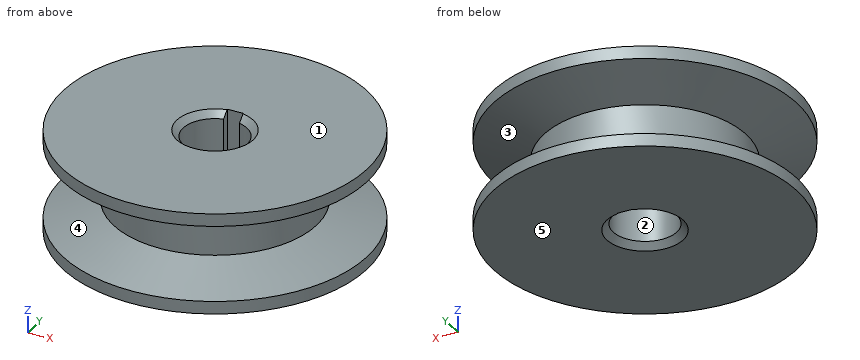
```python
from build123d import *

# Parameters (mm, degrees)
SKETCH1_R          = 19.05
SKETCH1_R_2        = 4
EXTRUDE1_DEPTH     = 6.35
CHAMFER1_SIZE      = 0.79375
SKETCH3_W          = 2
SKETCH3_H          = 2
CUT_EXTRUDE1_DEPTH = 30.784140075


with BuildPart() as part:
    # Sketch1 → Extrude1 (new, symmetric)
    with BuildSketch(Plane.XY):
        Circle(SKETCH1_R)
        Circle(SKETCH1_R_2, mode=Mode.SUBTRACT)
    extrude(amount=EXTRUDE1_DEPTH, both=True)

    # Chamfer1
    chamfer1_edges = [part.edges().sort_by_distance(p)[0] for p in [
        (-4, 0, -6.35),
        (-4, 0, 6.35),
    ]]
    chamfer(chamfer1_edges, length=CHAMFER1_SIZE)

    # Sketch2 → Cut-Revolve1 (revolve, cut)
    with BuildSketch(Plane(origin=(0, 0, 0), x_dir=(0, 0, -1), z_dir=(1, 0, 0)), mode=Mode.PRIVATE) as cut_revolve1_sk:
        Polygon((-4.7625, 19.05), (4.7625, 19.05), (2.451289012, 12.7), (-2.451289012, 12.7), align=None)
    revolve(cut_revolve1_sk.sketch.rotate(Axis((0, 0, 6.35), (0, 0, -1)), 180), axis=Axis((0, 0, 6.35), (0, 0, -1)), mode=Mode.SUBTRACT)

    # Sketch3 → Cut-Extrude1 (cut, through all)
    with BuildSketch(Plane.XY.offset(6.35)):
        with Locations((0, 3.8)):
            Rectangle(SKETCH3_W, SKETCH3_H)
    extrude(amount=-CUT_EXTRUDE1_DEPTH, mode=Mode.SUBTRACT)


solid = part.part
```
The model under review builds one solid part; all positions refer to its coordinate system, in mm. Face numbers are marked on the shaded views. A direction names the side the tool comes from. Give positions to 0.01 mm unless a question says otherwise; leave off trailing zeros. Write each loop counter-clockwise with the first axis right and the second up, starting at its lowest first coordinate (ties: lowest second). Pieces come first, ordered by that corner, then holes.
(1) Tool access review of the marked faces 4 and 5: name each direction out of +Z, -Z, +X, -X, +Y, -Y from which nothing blocks a thin tool from reaching the whole face with its end or side.
(2) For P1, Ø3, axis at y = -9.5, z = 0, coming from the -X side; P2, Ø2, axis at x = -0.5, z = 0.5, coming from the -Y side; P3, Ø5, axis at y = 4, z = 3.5, coming from the +X side; P4, Ø6.5, axis at x = 0, y = 0, coming from the -Z side, all flat-tipped, find the tip position at first contact; note any pin that passes through.
(3) To check wall thickness, follow L1, parallel to X at y = 0, z = 0.75; L2, parallel to Z at x = -3, y = 16.5; L3, parallel to Y at x = 2, z = -0.75. State the ranges of each line that lie inside material, in increasing order.
(4) Consider section C-C, the plane z = 0.75. Give the boundary of the cut face in (x, y).
(5) The part is to be moulded in two halves that separate along X. For the marked faces 1, 2 and 3, say which applies: released by +X, released by -X, zero draft, split by the parting line, or undercut.
(6) Consider section A-A, the plane y = 0. Give the boundary of the cut face in (x, z).
(7) Consider section B-B, the plane x = 0. Give the boundary of the cut face in (y, z), and give its area (3 significant figures).
Returned:
1. face 4: none
1. face 5: -Z, +X, -X, +Y, -Y
2. P1: stops at x = -9.86
2. P2: stops at y = -12.7
2. P3: stops at x = 18.96
2. P4: passes through
3. L1: x = -12.7 to -4, 4 to 12.7
3. L2: z = -6.35 to -3.93, 3.93 to 6.35
3. L3: y = -12.54 to -3.46, 3.46 to 12.54
4. outline: circle Ø25.4 at (0, 0); hole (-1, 3.87) arc R4 ccw (long way) to (1, 3.87) - (1, 4.8) - (-1, 4.8) - close
5. face 1: zero draft
5. face 2: undercut
5. face 3: split by the parting line
6. outline: (-19.05, -6.35) - (-4.79, -6.35) - (-4, -5.56) - (-4, 5.56) - (-4.79, 6.35) - (-19.05, 6.35) - (-19.05, 4.76) - (-12.7, 2.45) - (-12.7, -2.45) - (-19.05, -4.76) - close; (4, -5.56) - (4.79, -6.35) - (19.05, -6.35) - (19.05, -4.76) - (12.7, -2.45) - (12.7, 2.45) - (19.05, 4.76) - (19.05, 6.35) - (4.79, 6.35) - (4, 5.56) - close
7. outline: (-19.05, -6.35) - (-4.79, -6.35) - (-4, -5.56) - (-4, 5.56) - (-4.79, 6.35) - (-19.05, 6.35) - (-19.05, 4.76) - (-12.7, 2.45) - (-12.7, -2.45) - (-19.05, -4.76) - close; (4.8, -6.35) - (19.05, -6.35) - (19.05, -4.76) - (12.7, -2.45) - (12.7, 2.45) - (19.05, 4.76) - (19.05, 6.35) - (4.8, 6.35) - close
7. area: 280 mm2
